The listing builds one solid part. Answer for the finished solid, in the listing's coordinates (mm). Give positions to 0.01 mm unless a question says otherwise; leave off trailing zeros. Write each loop counter-clockwise with the first axis right and the second up, starting at its lowest first coordinate (ties: lowest second). Pieces come first, ordered by that corner, then holes.
```python
from build123d import *

# Parameters (mm, degrees)
EXTRUSION1_DEPTH           = 260
ESQUISSE2_R                = 1.5
EXTRUSION2_DEPTH           = 261.863949215
R_P_TITION_LIN_AIRE1_COUNT = 6
R_P_TITION_LIN_AIRE1_PITCH = 50
ESQUISSE3_R                = 1.5
EXTRUSION3_DEPTH           = 261.863949215
R_P_TITION_LIN_AIRE2_COUNT = 5
R_P_TITION_LIN_AIRE2_PITCH = 50


with BuildPart() as part:
    # Esquisse1 → Extrusion1 (new body)
    with BuildSketch(Plane.XY):
        Polygon((0, 0), (1.5, 0), (15, 0), (15, 1.5), (1.5, 1.5), (1.5, 15), (0, 15), align=None)
    extrude(amount=EXTRUSION1_DEPTH)

    # Esquisse2 → Extrusion2 (cut, through all)
    with BuildSketch(Plane.ZY):
        with Locations((5, 10)):
            Circle(ESQUISSE2_R)
    extrusion2 = extrude(amount=-EXTRUSION2_DEPTH, mode=Mode.SUBTRACT)

    # Répétition linéaire1: Extrusion2 ×6
    with Locations(*[(0, 0, i * R_P_TITION_LIN_AIRE1_PITCH) for i in range(1, R_P_TITION_LIN_AIRE1_COUNT)]):
        add(extrusion2, mode=Mode.SUBTRACT)

    # Esquisse3 → Extrusion3 (cut, through all)
    with BuildSketch(Plane.XZ):
        with Locations(Location((10, 30, 0), (0, 0, 270))):
            Circle(ESQUISSE3_R)
    extrusion3 = extrude(amount=-EXTRUSION3_DEPTH, mode=Mode.SUBTRACT)

    # Répétition linéaire2: Extrusion3 ×5
    with Locations(*[(0, 0, i * R_P_TITION_LIN_AIRE2_PITCH) for i in range(1, R_P_TITION_LIN_AIRE2_COUNT)]):
        add(extrusion3, mode=Mode.SUBTRACT)


solid = part.part
```
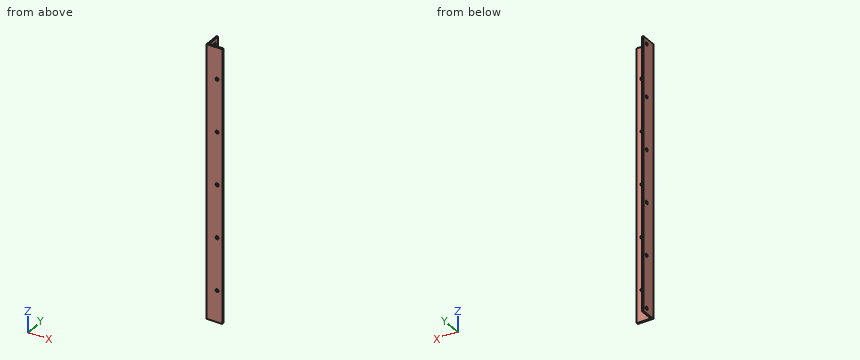
Item 1: Consider probe 1 along X at (y, z) = (0.6, 130); probe 2 along X at (y, z) = (14, 77.5). Determine where each line is inside the solid, lowest interval first.
Conclusion:
probe 1: x = 0 to 8.5, 11.5 to 15
probe 2: x = 0 to 1.5
Item 2: Each of these flat-tipped pins is pushed along its axis until it touches: P1, Ø1.8, axis at y = 10, z = 255, coming from the +X side; P2, Ø4, axis at y = 10, z = 105, coming from the +X side; P3, Ø1.5, axis at x = 2.5, z = 228.5, coming from the +Y side. Where does it stop, or does it pass through?
Conclusion:
P1: passes through
P2: stops at x = 1.5
P3: stops at y = 1.5
Item 3: A cutting plane is placed at A-A, the plane z = 167. Give the vertices of the cut face in (x, y).
Conclusion:
outline: (0, 0) - (15, 0) - (15, 1.5) - (1.5, 1.5) - (1.5, 15) - (0, 15) - close
Item 4: A cutting plane is placed at B-B, the plane x = 4. Give the vertices of the cut face in (y, z), plus the area to 3 significant figures.
Conclusion:
outline: (0, 0) - (1.5, 0) - (1.5, 260) - (0, 260) - close
area: 390 mm2
